from build123d import *

# Parameters (mm, degrees)
CYLINDER_R              = 2.8
CYLINDER_DEPTH          = 100
ARRAY_COUNT             = 3
CYLINDER001_R           = 5.5
CYLINDER001_DEPTH       = 38
CYLINDER001_PITCH_ANGLE = -90
SKETCH003_W             = 6
SKETCH003_H             = 20
POCKET_DEPTH            = 10
SKETCH002_R             = 4.2
PAD_DEPTH               = 38


with BuildPart() as set_screw_array:
    # Cylinder → Cylinder (new body)
    with BuildSketch(Plane(origin=(-33, 0, 0), x_dir=(1, 0, 0), z_dir=(0, 0, 1))):
        Circle(CYLINDER_R)
    extrude(amount=CYLINDER_DEPTH)

    # Array: Set Screw Array ×3 about axis
    array_axis = Axis((0, 0, 0), (1, 0, 0))


with BuildPart() as set_screw_array_1:
    add(set_screw_array.part)
    for i in range(1, ARRAY_COUNT):
        add(set_screw_array.part.rotate(array_axis, i * 360 / ARRAY_COUNT))


with BuildPart() as pocket:
    # Cylinder001 → Cylinder001 (new body)
    with BuildSketch(Plane.XY):
        Circle(CYLINDER001_R)
    extrude(amount=CYLINDER001_DEPTH)


with BuildPart() as pocket_1:
    # Cylinder001 pitch: moved
    add(pocket.part.rotate(Axis((0, 0, 0), (0, 1, 0)), CYLINDER001_PITCH_ANGLE))


with BuildPart() as pocket_2:
    # Cylinder001 placement: moved
    add(pocket_1.part)

    # Sketch003 → Pocket (cut)
    with BuildSketch(Plane.ZY.offset(38)):
        with Locations((7.1, 0)):
            Rectangle(SKETCH003_W, SKETCH003_H)
    extrude(amount=-POCKET_DEPTH, mode=Mode.SUBTRACT)


with BuildPart() as pad:
    # Sketch002 → Pad (new body)
    with BuildSketch(Plane.YZ):
        with Locations((0, 26.3725)):
            Circle(SKETCH002_R)
        with Locations((-22.839255, -13.18625)):
            Circle(SKETCH002_R)
        with Locations((22.839255, -13.18625)):
            Circle(SKETCH002_R)
    extrude(amount=-PAD_DEPTH)


with BuildPart() as cut002:
    # Sketch → Revolution (revolve)
    with BuildSketch(Plane.XY):
        Polygon((0, 37), (-13, 37), (-13, 14.2875), (-38, 14.2875), (-38, 0), (0, 0), align=None)
    revolve(axis=Axis((0, 0, 0), (1, 0, 0)))

    # Cut: cut Pad
    add(pad.part, mode=Mode.SUBTRACT)

    # Cut001: cut Pocket
    add(pocket_2.part, mode=Mode.SUBTRACT)

    # Cut002: cut Set Screw Array
    add(set_screw_array_1.part, mode=Mode.SUBTRACT)


solid = cut002.part
Geometry: final body of the model. Coordinates: model frame, mm. A direction names the side the tool comes from. Give positions to 0.01 mm unless a question says otherwise; leave off trailing zeros. Order: outer loops, then holes, each group sorted by start corner. A loop starts at its lowest first (then second) coordinate and runs counter-clockwise, first axis right, second up. Notation, with made-up numbers: (28, 63) -> (66, 63) arc R30 cw to (66, 101) -> close; hole circle Ø7 at (79.5, 78.5). An arc over 180 degrees is marked (long way). Put each result on its own line as item: value.
Q1. Section D-D, the plane x = -16. Return loops of the section in (y, z) (1 decimal).
Here are the results:
outline: circle Ø28.6 at (0, 0); hole circle Ø11 at (0, 0)
Q2. Section C-C, the plane z = 9. Return loops of the section in (x, y), then the cut area to 3 significant figures.
Here are the results:
outline: (-38, -11.1) -> (-13, -11.1) -> (-13, -35.89) -> (0, -35.89) -> (0, 35.89) -> (-13, 35.89) -> (-13, 11.1) -> (-38, 11.1) -> close; hole circle Ø5.6 at (-33, 0)
area: 1,460 mm^2
Q3. Draft query along X for faces 5 (the face through (-33, -3, 4.1)), 6 (the face through (0, -8, 1)), 7 (the face through (-33.365, 6.791, -7.126)). Return one class per face: released by +X, released by -X, zero draft, split by the parting line, or undercut.
Here are the results:
face 5: zero draft
face 6: released by +X
face 7: undercut
Q4. Section B-B, the plane x = -33. Return loops of the section in (y, z) (1 decimal).
Here are the results:
outline: (-13.5, -4.6) -> (-5.5, 0.1) arc R5.5 cw to (-3.7, 4.1) -> (-2.8, 4.1) -> (-2.8, 14) arc R14.3 ccw to start; (-10.7, -9.4) arc R14.3 ccw to (10.7, -9.4) -> (2.7, -4.8) arc R5.5 cw to (-2.7, -4.8) -> close; (2.8, 4.1) -> (3.7, 4.1) arc R5.5 cw to (5.5, 0.1) -> (13.5, -4.6) arc R14.3 ccw to (2.8, 14) -> close
Q5. Pin query (flat end, axial travel): pin 1 (6 mm diameter, centred on x = -28.5, z = 13.5, fed in from -Y); pin 2 (4 mm diameter, centred on x = -25.5, z = 10.5, fed in from -Y); pin 3 (2 mm diameter, centred on x = -34.5, y = -0.5, fed in from -Z). Return the tip coordinate at first contact, or that it passes through.
Here are the results:
pin 1: stops at y = -9.69
pin 2: stops at y = -11.48
pin 3: stops at z = -14.29
Q6. Material intervals for L1, parallel to Z at x = -8, y = 0; L2, parallel to Z at x = -14, y = 0; L3, parallel to Z at x = -3.5, y = -2, sorted ascending.
Here are the results:
L1: z = -37 to -5.5, 5.5 to 22.17, 30.57 to 37
L2: z = -14.29 to -5.5, 5.5 to 14.29
L3: z = -36.95 to -5.12, 5.12 to 22.68, 30.07 to 36.95
Q7. Section A-A, the plane y = 0. Return loops of the section in (x, z), then the cut area to 3 significant figures.
Here are the results:
outline: (-38, -14.29) -> (-13, -14.29) -> (-13, -37) -> (0, -37) -> (0, -5.5) -> (-38, -5.5) -> close; (-38, 4.1) -> (-35.8, 4.1) -> (-35.8, 14.29) -> (-38, 14.29) -> close; (-30.2, 4.1) -> (-28, 4.1) -> (-28, 5.5) -> (0, 5.5) -> (0, 22.17) -> (-13, 22.17) -> (-13, 14.29) -> (-30.2, 14.29) -> close; (-13, 30.57) -> (0, 30.57) -> (0, 37) -> (-13, 37) -> close
area: 1,110 mm^2
Q8. Reachability of faces 1 (the face through (-35.8, 0.1, 9.1)), 2 (the face through (-13, 16, 1)), 3 (the face through (-38, 0, -6)), 4 (the face through (-18.734, 0.242, -5.495)) from +Z, -Z, +X, -X, +Y, -Y: full face, straight path, thin tool, end or side. Return the list, or none.
Here are the results:
face 1: +Z
face 2: -X
face 3: +Z, -Z, -X, +Y, -Y
face 4: +X
